Geometry: final body of the model. Coordinates: model frame, mm. A direction names the side the tool comes from. Give positions to 0.01 mm unless a question says otherwise; leave off trailing zeros. Write each loop counter-clockwise with the first axis right and the second up, starting at its lowest first coordinate (ties: lowest second). Pieces come first, ordered by that corner, then holes.
from build123d import *

# Parameters (mm, degrees)
SKETCH1_W                         = 165.1
SKETCH1_H                         = 64
BOSS_EXTRUDE1_DEPTH               = 9.525
F_1_4_CLEARANCE_HOLE1_D           = 6.7564
F_1_4_CLEARANCE_HOLE1_CSINK_D     = 8.0264
F_1_4_CLEARANCE_HOLE1_CSINK_ANGLE = 100
CBORE_FOR_M5_SHCS1_AT_2_COUNT     = 2
CBORE_FOR_M5_SHCS1_AT_2_PITCH     = 44
CBORE_FOR_M5_SHCS1_AT_3_COUNT     = 2
CBORE_FOR_M5_SHCS1_AT_3_PITCH     = 50.119856345
CBORE_FOR_M5_SHCS1_AT_4_COUNT     = 2
CBORE_FOR_M5_SHCS1_AT_4_PITCH     = 24


with BuildPart() as part:
    # Sketch1 → Boss-Extrude1 (new body)
    with BuildSketch(Plane(origin=(0, 0, 0), x_dir=(1, 0, 0), z_dir=(0, 1, 0))):
        with Locations((82.55, 32)):
            Rectangle(SKETCH1_W, SKETCH1_H)
    extrude(amount=BOSS_EXTRUDE1_DEPTH)

    # 1/4 Clearance Hole1 (through all)
    with Locations(Plane(origin=(0, 9.525, 0), x_dir=(1, 0, 0), z_dir=(0, 1, 0))):
        with Locations((152.4, 51.3), (152.4, 12.7)):
            CounterSinkHole(F_1_4_CLEARANCE_HOLE1_D / 2, F_1_4_CLEARANCE_HOLE1_CSINK_D / 2, counter_sink_angle=F_1_4_CLEARANCE_HOLE1_CSINK_ANGLE)

    # Sketch7 → CBORE for M5 SHCS1 (revolve, cut)
    with BuildSketch(Plane(origin=(6, 0, -44), x_dir=(0, 0, -1), z_dir=(1, 0, 0))):
        Polygon((0, 0), (0, 9.525), (2.75, 9.525), (2.75, 5), (5, 5), (5, 0.020977491), (5.025, 0), align=None)
    cbore_for_m5_shcs1 = revolve(axis=Axis((6, -6.35, -44), (0, 1, 0)), mode=Mode.SUBTRACT)

    # CBORE for M5 SHCS1 at 2: CBORE for M5 SHCS1 ×2
    with Locations(*[(i * CBORE_FOR_M5_SHCS1_AT_2_PITCH, 0, 0) for i in range(1, CBORE_FOR_M5_SHCS1_AT_2_COUNT)]):
        add(cbore_for_m5_shcs1, mode=Mode.SUBTRACT)

    # CBORE for M5 SHCS1 at 3: CBORE for M5 SHCS1 ×2
    with Locations(*[Vector(0.8778955729143844, 0, 0.4788521306805733) * (i * CBORE_FOR_M5_SHCS1_AT_3_PITCH) for i in range(1, CBORE_FOR_M5_SHCS1_AT_3_COUNT)]):
        add(cbore_for_m5_shcs1, mode=Mode.SUBTRACT)

    # CBORE for M5 SHCS1 at 4: CBORE for M5 SHCS1 ×2
    with Locations(*[(0, 0, i * CBORE_FOR_M5_SHCS1_AT_4_PITCH) for i in range(1, CBORE_FOR_M5_SHCS1_AT_4_COUNT)]):
        add(cbore_for_m5_shcs1, mode=Mode.SUBTRACT)


solid = part.part
Q1. Access query for faces 5 (the flat face through (52.2, 5, -17.8)), 6 (the flat face through (81, 9.525, -32)). Directions: +Z, -Z, +X, -X, +Y, -Y. A direction counts if a zero-diameter tool reaches every point of the face in a straight line with its end or side. Return the directions, or none.
Filled sheet:
face 5: -Y
face 6: +Z, -Z, +X, -X, +Y
Q2. Section D-D on z = -44. Output: boundary loops of the cut face in (x, y) (3 decimals).
Filled sheet:
outline: (0, 0) - (0.975, 0) - (1, 0.021) - (1, 5) - (3.25, 5) - (3.25, 9.525) - (0, 9.525) - close; (8.75, 5) - (11, 5) - (11, 0.021) - (11.025, 0) - (44.975, 0) - (45, 0.021) - (45, 5) - (47.25, 5) - (47.25, 9.525) - (8.75, 9.525) - close; (52.75, 5) - (55, 5) - (55, 0.021) - (55.025, 0) - (165.1, 0) - (165.1, 9.525) - (52.75, 9.525) - close
Q3. Section A-A on x = 6. Output: boundary loops of the cut face in (y, z) (3 decimals), plus the area to 3 significant figures.
Filled sheet:
outline: (0, -64) - (9.525, -64) - (9.525, -46.75) - (5, -46.75) - (5, -49) - (0.021, -49) - (0, -49.025) - close; (0, -38.975) - (0.021, -39) - (5, -39) - (5, -41.25) - (9.525, -41.25) - (9.525, -22.75) - (5, -22.75) - (5, -25) - (0.021, -25) - (0, -25.025) - close; (0, -14.975) - (0.021, -15) - (5, -15) - (5, -17.25) - (9.525, -17.25) - (9.525, 0) - (0, 0) - close
area: 460 mm2
Q4. Pull-direction query (Z, two-part tool) for faces 1 (the cylindrical face through (48.141, 7.231, -41.973)), 2 (the flat face through (0, 5, -32)), 3 (the cylindrical face through (6, 2, -39)), 4 (the flat face through (81, 5, 0)); classes: released by +Z, released by -Z, zero draft, split by the parting line, or undercut.
Filled sheet:
face 1: undercut
face 2: zero draft
face 3: undercut
face 4: released by +Z
Q5. Section B-B on z = -51.3. Output: boundary loops of the cut face in (x, y) (3 decimals), plus the area to 3 significant figures.
Filled sheet:
outline: (0, 0) - (149.022, 0) - (149.022, 8.992) - (148.387, 9.525) - (0, 9.525) - close; (155.778, 0) - (165.1, 0) - (165.1, 9.525) - (156.413, 9.525) - (155.778, 8.992) - close
area: 1,510 mm2
Q6. Section C-C on y = 1.5. Output: boundary loops of the cut face in (x, z).
Filled sheet:
outline: (0, -64) - (165.1, -64) - (165.1, 0) - (0, 0) - close; hole circle Ø10 at (6, -44); hole circle Ø10 at (6, -20); hole circle Ø10 at (50, -44); hole circle Ø10 at (50, -20); hole circle Ø6.76 at (152.4, -51.3); hole circle Ø6.76 at (152.4, -12.7)
Q7. Ray query, line 1 along X through (y, z) = (7.3, -44); line 2 along Z through (x, y) = (152.4, 2.25); line 3 along Z through (x, y) = (6, 6.2). Return the intervals inside material, ascending.
Filled sheet:
line 1: x = 0 to 3.25, 8.75 to 47.25, 52.75 to 165.1
line 2: z = -64 to -54.68, -47.92 to -16.08, -9.32 to 0
line 3: z = -64 to -46.75, -41.25 to -22.75, -17.25 to 0
